The listing builds one solid part. Answer for the finished solid, in the listing's coordinates (mm). Coordinates: 2 decimals unless noted, no trailing zeros. Loops run counter-clockwise (first coordinate to the right, second up) from the corner with the lowest first, then second, coordinate; pieces in that order, holes last. Notation, with made-up numbers: (22.25, 63) - (46.25, 63) arc R32 cw to (46.25, 98) - close; hole circle Ø5 at (1.5, -18). An arc over 180 degrees is marked (long way). Write each question's results on one line, items separated by ' | '. Start each with the question number.
(1) Find section A-A on z = -13. Determine the outline of the cut face in (x, y), then the cut area to 3 significant figures.
(2) Consider line 1 (Z direction, x = 1, y = 15); line 2 (X direction, y = 20.25, z = -7); line 3 (Z direction, x = -6, y = 7). Determine where each line is inside the solid, lowest interval first. Write a range as from..to.
(3) Find section B-B on x = 11.75. Determine the outline of the cut face in (y, z).
(4) Given pin 1 Ø3 at (x, z) = (-7.5, -7) entering from +Y; pin 2 Ø4 at (y, z) = (10, -12.5) entering from +X, each flat-ended and moving along its own axis, determine where each tip first touches the part or whether it passes through.
Autodesk Inventor part; units mm, degrees
ref_plane "YZ Plane" through (0, 0, 0) normal (1, 0, 0) x (0, 1, 0)
ref_plane "XZ Plane" through (0, 0, 0) normal (0, 1, 0) x (-1, 0, 0)
ref_plane "XY Plane" through (0, 0, 0) normal (0, 0, 1) x (1, 0, 0)
sketch "Sketch1" plane through (0, 0, 0) normal (0, 1, 0) x (-1, 0, 0)
  line L0 (0, 0) -> (15, 0)
  line L1 (15, 0) -> (15, -15)
  line L2 (15, -15) -> (0, -15)
  line L3 (0, -15) -> (0, 0)
  circle A0 centre (7.5, -7.5) radius 4.3
  dimension "soporte_largo" = 15
  dimension "soporte_ancho" = 15
  dimension "soporte_hueco_diametro" = 8.6
  dimension "soporte_hueco_pos_ancho" = 7.5
  dimension "soporte_hueco_pos_largo" = 7.5
sketch "Sketch2" plane through (0, 0, 0) normal (0, 0, 1) x (1, 0, 0)
  line L0 (0, 0) -> (14.4338, 25)
  line L1 (0, 0) -> (28.8675, 0) construction
  dimension "soporte_inclinacion" = 60
  dimension "soporte_alterura" = 25
sweep "Sweep1" add profiles "Sketch1" path "Sketch2"
equation "\"soporte_hueco_pos_ancho\" = 0.5 * soporte_ancho"
equation "\"soporte_hueco_pos_largo\" = 0.5 * soporte_largo"
equation "\"tol1\" = 0.1"
equation "\"tol2\" = 0.2"
equation "\"tol3\" = 0.3"
equation "\"tol4\" = 0.4"
equation "\"tol5\" = 0.5"
equation "\"tol6\" = 0.6"
equation "\"tol7\" = 0.7"
equation "\"tol8\" = 0.8"
equation "\"tol9\" = 0.9"
equation "\"tol\" = 7"
properties part number "TestSoporte"
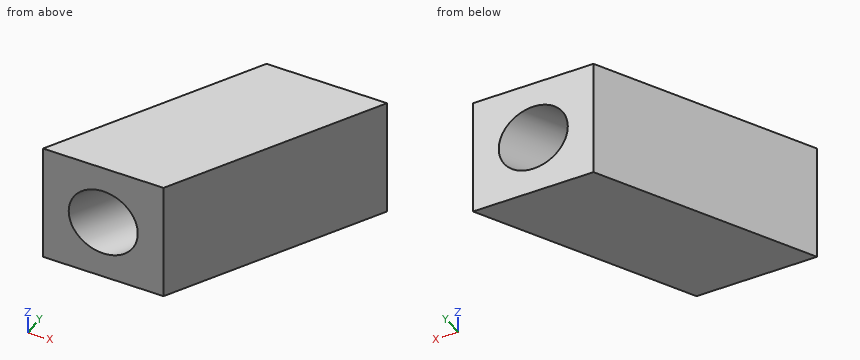
Values:
1) outline: (-15, 0) - (0, 0) - (14.43, 25) - (-0.57, 25) - close | area: 375 mm²
2) line 1: z = -15..-11.8, -3.2..0 | line 2: x = -3.31..-0.08, 8.46..11.69 | line 3: z = -15..-10.97, -4.03..0
3) outline: (20.35, -15) - (25, -15) - (25, 0) - (20.35, 0) - close
4) pin 1: stops at y = 15.59 | pin 2: stops at x = 6.93
